Input: part model. Units: mm. Frame: model coordinates. Face numbers are marked on the shaded views. A direction names the side the tool comes from. Coordinates: 2 decimals unless noted, no trailing zeros. Write each loop counter-clockwise with the first axis right and the second up, starting at its lowest first coordinate (ties: lowest second). Pieces come first, ordered by that corner, then holes. Notation, with made-up numbers: M 29,27.25 L 49,27.25 A16 ccw 49,36.25 Z; hole C 60,-27.5 d1. An arc over 180 degrees is marked long. Write each question's results on one line, items separated by ' | '. Start each with the question number.
1. First-contact query: pin 1 (3 mm diameter, centred on y = 22, z = -1, fed in from +X); pin 2 (2 mm diameter, centred on y = 23, z = -2.5, fed in from -X); pin 3 (8 mm diameter, centred on x = 2.5, z = -3, fed in from +Y); pin 4 (10 mm diameter, centred on y = 19.5, z = -7.5, fed in from +X). Flat tips, straight axial feed; report the tip coordinate or a pass-through.
2. Section query B-B, the plane y = 21.5. Output: boundary loops of the cut face in (x, z), and give its area (3 significant figures).
3. Set-up query: the marked faces 1 and 2. Return all of +Z, -Z, +X, -X, +Y, -Y with unobstructed straight access to the full face (end or side cutting, diameter ignored); none if empty.
4. Pull-direction query (Z, two-part tool) for the marked faces 3, 4 and 5; classes: +Z half, -Z half, draft (parallel to the pull), parting line (faces both ways), or undercut.
5. Section query C-C, the plane x = 1.25. Count the separate pieces of the cut face and the enclosed holes in it, and give its area (3 significant figures).
6. Ray query, probe 1 along Y at (x, z) = (-4, -1); probe 2 along X at (y, z) = (1.55, 9); probe 3 along Z at (x, y) = (3, 3.5). Return the intervals inside material, ascending.
7. Section query A-A, the plane z = 9. Output: boundary loops of the cut face in (x, y).
```python
from build123d import *

# Parameters (mm, degrees)
SKETCH1_W               = 15
SKETCH1_H               = 27
SKETCH1_R               = 1.6
BOSS_EXTRUDE1_DEPTH     = 3
SKETCH2_W               = 4
SKETCH2_H               = 27
BOSS_EXTRUDE2_DEPTH     = 23
SKETCH3_W               = 27
SKETCH3_H               = 2
CUT_EXTRUDE1_DEPTH      = 1
SKETCH4_W               = 27
SKETCH4_H               = 2.6
CUT_EXTRUDE2_DEPTH      = 1
SKETCH5_W               = 11
SKETCH5_H               = 2
BOSS_EXTRUDE3_DEPTH     = 17
CUT_EXTRUDE3_DEPTH      = 37.84087404
CUT_EXTRUDE3_DEPTH_BACK = 37.84087404
SKETCH7_RX              = 17
SKETCH7_RY              = 11
FILLET2_R               = 1
FILLET3_START           = -11.5
FILLET3_DEPTH           = 23
FILLET3_START_2         = 2
FILLET3_2_DEPTH         = 18
FILLET3_3_DEPTH         = 23


with BuildPart() as part:
    # Sketch1 → Boss-Extrude1 (new body)
    with BuildSketch(Plane(origin=(0, 0, 0), x_dir=(1, 0, 0), z_dir=(0, 1, 0))):
        Rectangle(SKETCH1_W, SKETCH1_H)
        with Locations(Location((2.5, 9, 0), (0, 0, 270))):
            Circle(SKETCH1_R, mode=Mode.SUBTRACT)
        with Locations(Location((2.5, -9, 0), (0, 0, 90))):
            Circle(SKETCH1_R, mode=Mode.SUBTRACT)
    extrude(amount=BOSS_EXTRUDE1_DEPTH)

    # Sketch2 → Boss-Extrude2 (add)
    with BuildSketch(Plane(origin=(0, 3, 0), x_dir=(1, 0, 0), z_dir=(0, 1, 0))):
        with Locations((-5.5, 0)):
            Rectangle(SKETCH2_W, SKETCH2_H)
    extrude(amount=BOSS_EXTRUDE2_DEPTH)

    # Sketch3 → Cut-Extrude1 (cut)
    with BuildSketch(Plane.ZY.offset(7.5)):
        with Locations((0, 23.2)):
            Rectangle(SKETCH3_W, SKETCH3_H)
    extrude(amount=-CUT_EXTRUDE1_DEPTH, mode=Mode.SUBTRACT)

    # Sketch4 → Cut-Extrude2 (cut)
    with BuildSketch(Plane(origin=(-3.5, 0, 0), x_dir=(0, 0, -1), z_dir=(1, 0, 0))):
        with Locations((0, 21.3)):
            Rectangle(SKETCH4_W, SKETCH4_H)
    extrude(amount=-CUT_EXTRUDE2_DEPTH, mode=Mode.SUBTRACT)

    # Sketch5 → Boss-Extrude3 (add)
    with BuildSketch(Plane(origin=(0, 3, 0), x_dir=(1, 0, 0), z_dir=(0, 1, 0))):
        with Locations((2, 12.5)):
            Rectangle(SKETCH5_W, SKETCH5_H)
        with Locations((2, -12.5)):
            Rectangle(SKETCH5_W, SKETCH5_H)
    extrude(amount=BOSS_EXTRUDE3_DEPTH)

    # Sketch7 → Cut-Extrude3 (cut, two sides: drawn at the far end of the back side and taken through both)
    with BuildSketch(Plane.XY.offset(-11.5).offset(-CUT_EXTRUDE3_DEPTH_BACK)):
        with Locations(Location((7.5, 20), (0, 0, 90))):
            Ellipse(SKETCH7_RX, SKETCH7_RY)
    extrude(amount=CUT_EXTRUDE3_DEPTH + CUT_EXTRUDE3_DEPTH_BACK, mode=Mode.SUBTRACT)

    # Fillet2
    fillet2_edges = [part.edges().sort_by_distance(p)[0] for p in [
        (-7.5, 25.1, 13.5),
        (-7.5, 11.1, 13.5),
        (7.5, 1.5, 13.5),
        (-4.5, 21.3, 13.5),
        (-3.5, 24.3, 13.5),
        (-7.5, 25.1, -13.5),
        (-7.5, 11.1, -13.5),
        (7.5, 1.5, -13.5),
        (-4.5, 21.3, -13.5),
        (-3.5, 24.3, -13.5),
    ]]
    fillet(fillet2_edges, radius=FILLET2_R - 0.0001)  # a hair under: the kernel refuses the full size

    # Fillet3: read off the stored shape, not the designer's step
    # Fillet3 outline → Fillet3 (add)
    with BuildSketch(Plane.XY.offset(FILLET3_START)):
        with BuildLine():
            ThreePointArc((-2.5, 3), (-3.207106781, 3.292893219), (-3.5, 4))
            Line((-3.5, 4), (-3.5, 3))
            Line((-3.5, 3), (-2.5, 3))
        make_face()
    extrude(amount=FILLET3_DEPTH)

    # Fillet3 2 outline → Fillet3 2 (add)
    with BuildSketch(Plane(origin=(0, 0, 0), x_dir=(1, 0, 0), z_dir=(0, 1, 0)).offset(FILLET3_START_2)):
        with BuildLine():
            Line((-3.5, 11.5), (-3.5, 10.5))
            ThreePointArc((-3.5, 10.5), (-3.207106781, 11.207106781), (-2.5, 11.5))
            Line((-2.5, 11.5), (-3.5, 11.5))
        make_face()
        with BuildLine():
            ThreePointArc((-2.5, -11.5), (-3.207106781, -11.207106781), (-3.5, -10.5))
            Line((-3.5, -10.5), (-3.5, -11.5))
            Line((-3.5, -11.5), (-2.5, -11.5))
        make_face()
    extrude(amount=FILLET3_2_DEPTH)

    # Fillet3 3 outline → Fillet3 3 (cut)
    with BuildSketch(Plane.XY.offset(FILLET3_START)):
        with BuildLine():
            Line((-2.5, 20), (-3.5, 20))
            add(Edge.make_bspline(
                [(-3.5, 20), (-3.5, 16.290295866), (-2.5, 12.917837562)],
                knots=[4.71238898, 4.71238898, 4.71238898, 5.142088647, 5.142088647, 5.142088647], degree=2, weights=[1, 0.977008421, 1]))
            Line((-2.5, 12.917837562), (-2.5, 20))
        make_face()
    extrude(amount=FILLET3_3_DEPTH, mode=Mode.SUBTRACT)


solid = part.part
```
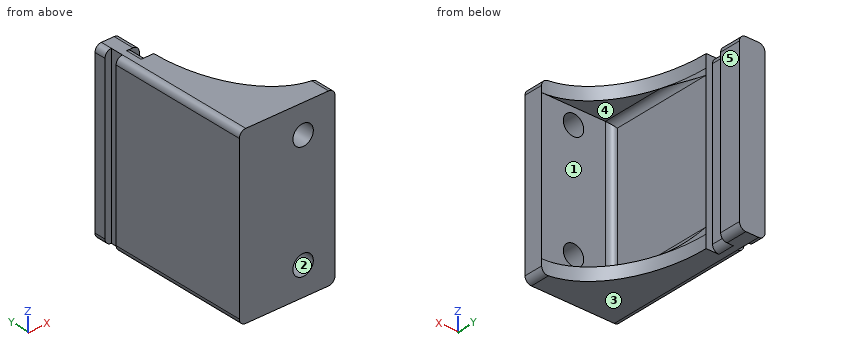
Answer:
1) pin 1: x = -3.5 | pin 2: x = -7.5 | pin 3: y = 3 | pin 4: x = -3.21
2) outline: M -7.5,-12.5 A1 ccw -6.5,-13.5 L -5.5,-13.5 A1 ccw -4.5,-12.5 L -4.5,12.5 A1 ccw -5.5,13.5 L -6.5,13.5 A1 ccw -7.5,12.5 Z | area: 80.1 mm^2
3) face 1: +X, +Y | face 2: +Y, -Y
4) face 3: -Z half | face 4: undercut | face 5: draft
5) separate pieces: 3 | enclosed holes: 0 | area: 81.1 mm^2
6) probe 1: 0 to 20, 22.6 to 26 | probe 2: -7.5 to 0.9, 4.1 to 7.5 | probe 3: -13.5 to -11.5, 11.5 to 13.5
7) outline: M -7.5,0 L 0.9,0 L 0.9,3 L -2.5,3 A1 cw -3.5,4 L -3.5,20 L -4.5,20 L -4.5,22.6 L -3.5,22.6 L -3.5,26 L -7.5,26 L -7.5,24.2 L -6.5,24.2 L -6.5,22.2 L -7.5,22.2 Z; M 4.1,0 L 7.5,0 L 7.5,3 L 4.1,3 Z
